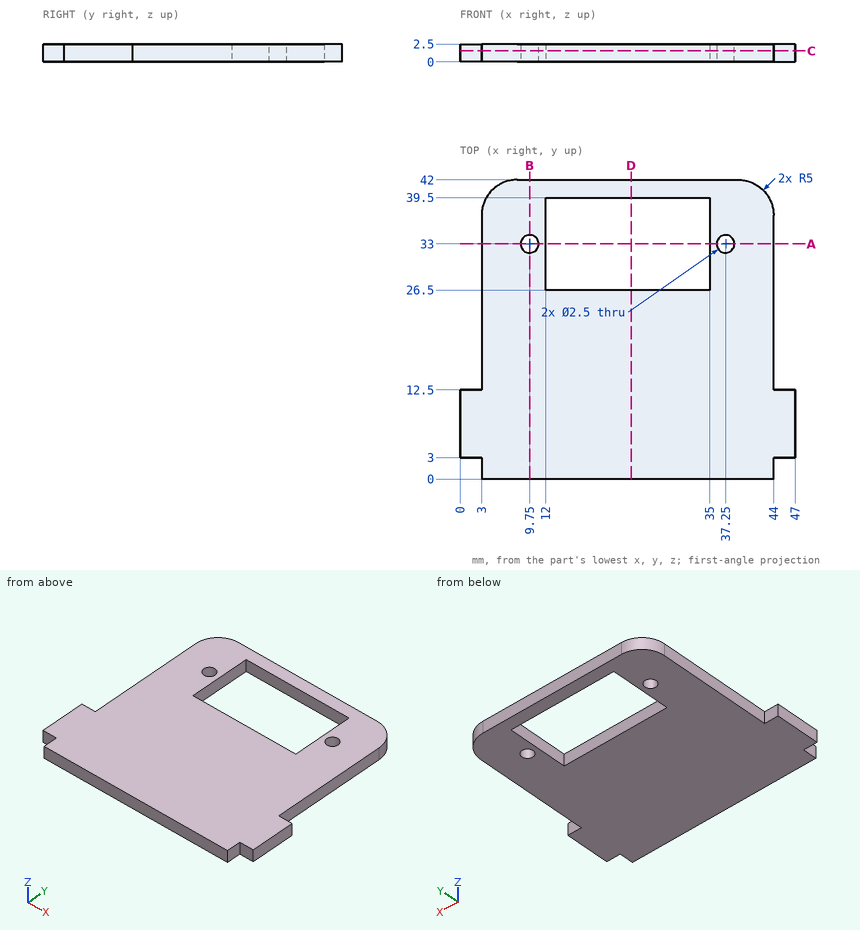
Geometry: see drawing. Coordinates: mm, zero at the bounding-box minimum. Coordinates: 2 decimals unless noted, no trailing zeros. Loops run counter-clockwise (first coordinate to the right, second up) from the corner with the lowest first, then second, coordinate; pieces in that order, holes last.
Q1. Contact query for flat-ended pins moving along their axis: pin 1 (0.8 mm diameter, centred on y = 31.5, z = 2, fed in from -X); pin 2 (0.8 mm diameter, centred on x = 46, z = 1, fed in from -Y); pin 3 (1.2 mm diameter, centred on x = 45, z = 1, fed in from +Y). Output: stop coordinate, or through.
Q2. Cut plane D-D (x = 24). Output: boundary loops of the cut face in (y, z).
Q3. Cut plane C-C (z = 1.55). Output: boundary loops of the cut face in (x, y).
Q4. Material intervals for line 1 (X direction, y = 33, z = 0.5); line 2 (Y direction, x = 37.25, z = 0.85); line 3 (X direction, y = 33.5, z = 0.3), sorted ascending.
Q5. Cut plane B-B (x = 9.75). Output: boundary loops of the cut face in (y, z).
Q6. Cut plane A-A (y = 33). Output: boundary loops of the cut face in (x, z).
Working result:
1. pin 1: stops at x = 3
1. pin 2: stops at y = 3
1. pin 3: stops at y = 12.5
2. outline: (0, 0) - (26.5, 0) - (26.5, 2.5) - (0, 2.5) - close; (39.5, 0) - (42, 0) - (42, 2.5) - (39.5, 2.5) - close
3. outline: (0, 3) - (3, 3) - (3, 0) - (44, 0) - (44, 3) - (47, 3) - (47, 12.5) - (44, 12.5) - (44, 37) arc R5 ccw to (39, 42) - (8, 42) arc R5 ccw to (3, 37) - (3, 12.5) - (0, 12.5) - close; hole circle Ø2.5 at (9.75, 33); hole (12, 26.5) - (35, 26.5) - (35, 39.5) - (12, 39.5) - close; hole circle Ø2.5 at (37.25, 33)
4. line 1: x = 3 to 8.5, 11 to 12, 35 to 36, 38.5 to 44
4. line 2: y = 0 to 31.75, 34.25 to 42
4. line 3: x = 3 to 8.6, 10.9 to 12, 35 to 36.1, 38.4 to 44
5. outline: (0, 0) - (31.75, 0) - (31.75, 2.5) - (0, 2.5) - close; (34.25, 0) - (42, 0) - (42, 2.5) - (34.25, 2.5) - close
6. outline: (3, 0) - (8.5, 0) - (8.5, 2.5) - (3, 2.5) - close; (11, 0) - (12, 0) - (12, 2.5) - (11, 2.5) - close; (35, 0) - (36, 0) - (36, 2.5) - (35, 2.5) - close; (38.5, 0) - (44, 0) - (44, 2.5) - (38.5, 2.5) - close
